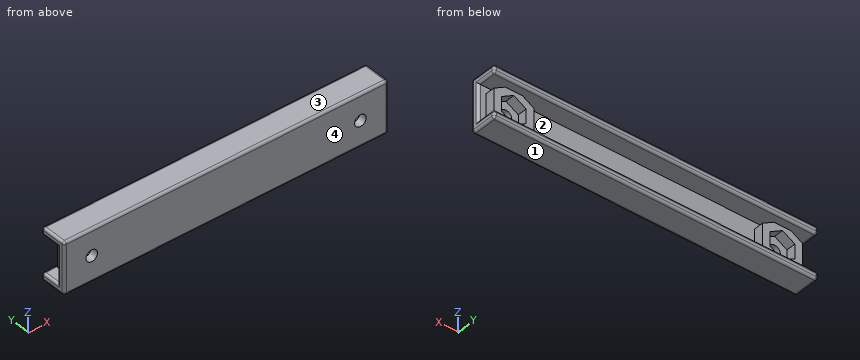
Autodesk Inventor part; units mm, degrees
ref_plane "YZ Plane" through (0, 0, 0) normal (1, 0, 0) x (0, 1, 0)
ref_plane "XZ Plane" through (0, 0, 0) normal (0, 1, 0) x (-1, 0, 0)
ref_plane "XY Plane" through (0, 0, 0) normal (0, 0, 1) x (1, 0, 0)
sketch "Sketch1" plane through (0, 0, 0) normal (0, 1, 0) x (-1, 0, 0)
  line L0 (0, 0) -> (107.315, 0)
  line L1 (107.315, 0) -> (107.315, -17.145)
  line L2 (107.315, 0) -> (124.46, 0) construction
  line L3 (107.315, -17.145) -> (0, -17.145)
  line L4 (0, -17.145) -> (0, 0)
  dimension "d0" = 107.315
  dimension "d1" = 17.145
  dimension "d2" = 90
extrude "Extrusion1" add sketch "Sketch1" along normal blind 2.54
sketch "Sketch2" plane through (0, 2.54, 0) normal (0, 1, 0) x (1, 0, 0)
  line L0 (0, 0) -> (0, 17.145)
  line L1 (0, 8.5725) -> (-9.2075, 8.5725) construction
  line L2 (0, 8.5725) -> (-2.576, 8.5725)
  line L3 (-2.576, 8.5725) -> (-2.576, 12.4012)
  line L4 (-2.576, 8.5725) -> (-2.576, 4.7438)
  line L5 (0, 17.145) -> (0, 14.605)
  line L6 (0, 14.605) -> (-107.315, 14.605)
  line L7 (-107.315, 17.145) -> (-107.315, 0)
  line L8 (-107.315, 14.605) -> (-107.315, 17.145)
  line L9 (0, 17.145) -> (-107.315, 17.145)
  line L10 (-107.315, 17.145) -> (0, 17.145)
  line L11 (0, 0) -> (0, 2.54)
  line L12 (0, 2.54) -> (-107.315, 2.54)
  line L13 (-107.315, 0) -> (0, 0)
  line L14 (-2.576, 12.4012) -> (-6.3932, 14.605)
  line L15 (-6.3932, 14.605) -> (-12.032, 14.605)
  line L16 (-2.576, 4.7438) -> (-6.3932, 2.54)
  line L17 (-12.032, 14.605) -> (-15.839, 12.4071)
  line L18 (-15.839, 12.4071) -> (-15.839, 4.7438)
  line L19 (-15.839, 4.7438) -> (-12.0218, 2.54)
  line L20 (-9.2075, 13.2969) -> (-5.116, 10.9347)
  line L21 (-5.116, 10.9347) -> (-5.116, 6.2103)
  line L22 (-5.116, 6.2103) -> (-9.2075, 3.8481)
  line L23 (-9.2075, 3.8481) -> (-13.299, 6.2103)
  line L24 (-13.299, 6.2103) -> (-13.299, 10.9347)
  line L25 (-13.299, 10.9347) -> (-9.2075, 13.2969)
  line L26 (-53.6575, 14.605) -> (-53.6575, 2.54) construction
  line L27 (-107.315, 8.5725) -> (-98.1075, 8.5725) construction
  line L28 (-107.315, 8.5725) -> (-104.739, 8.5725)
  line L29 (-104.739, 8.5725) -> (-104.739, 12.4012)
  line L30 (-104.739, 8.5725) -> (-104.739, 4.7438)
  line L31 (-104.739, 12.4012) -> (-100.9218, 14.605)
  line L32 (-104.739, 4.7438) -> (-100.9218, 2.54)
  line L33 (-95.283, 14.605) -> (-91.476, 12.4071)
  line L34 (-91.476, 12.4071) -> (-91.476, 4.7438)
  line L35 (-91.476, 4.7438) -> (-95.2932, 2.54)
  line L36 (-98.1075, 8.5725) -> (-98.1075, 14.605)
  line L37 (-98.1075, 13.2969) -> (-102.199, 10.9347)
  line L38 (-102.199, 10.9347) -> (-102.199, 6.2103)
  line L39 (-102.199, 6.2103) -> (-98.1075, 3.8481)
  line L40 (-98.1075, 3.8481) -> (-94.016, 6.2103)
  line L41 (-94.016, 6.2103) -> (-94.016, 10.9347)
  line L42 (-94.016, 10.9347) -> (-98.1075, 13.2969)
  line L43 (-100.9218, 14.605) -> (-95.283, 14.605)
  line L44 (-100.9218, 2.54) -> (-95.2932, 2.54)
  point P0 (-8.3776, 2.54)
  point P1 (-9.2075, 14.605)
  dimension "d5" = 9.2075
  dimension "d16" = 2.54
  dimension "d17" = 90
  dimension "d18" = 2.54
  dimension "d20" = 5.6388
  dimension "d30" = 4.7244
  dimension "d43" = 2.54
  dimension "d44" = 2.54
  dimension "d45" = 2.54
  dimension "d46" = 2.54
hole "Hole1" at (-9.2075, 2.54, -8.5725) direction (0, -1, 0) diameter 3.81 end through all
extrude "Extrusion2" add sketch "Sketch2" along normal blind 6.35 contours L13 L7 L12 L0 | L6 L7 L9 L0
extrude "Extrusion4" add sketch "Sketch2" along normal blind 3.175 contours L12 L19 L18 L17 L6 L14 L3 L4 L16 | L32 L30 L29 L31 L6 L33 L34 L35 L12
hole "Hole2" at (-98.1075, 2.54, -8.5725) direction (0, -1, 0) diameter 3.81 end through all
fillet "Fillet1" radius 0.7874 22 edges at (-107.315, 0, -8.5725) (-53.6575, 0, 0) (-53.6575, 0, -17.145) (0, 0, -8.5725) (-107.315, 4.445, -17.145) (-107.315, 5.715, -14.605) (-107.315, 2.54, -8.5725) (-107.315, 5.715, -2.54) (-107.315, 4.445, 0) (-107.315, 8.89, -1.27) (-107.315, 8.89, -15.875) (-53.6575, 8.89, -17.145) (-53.6575, 8.89, -14.605) (-53.6575, 8.89, -2.54) (-53.6575, 8.89, 0) (0, 8.89, -1.27) (0, 4.445, 0) (0, 5.715, -2.54) (0, 2.54, -8.5725) (0, 5.715, -14.605) (0, 4.445, -17.145) (0, 8.89, -15.875)
equation "\"BendRadius\" = Thickness"
equation "\"BendReliefWidth\" = Thickness"
equation "\"BendReliefDepth\" = 0.5 * Thickness"
equation "\"CornerReliefSize\" = 4 * Thickness"
equation "\"MinimumRemnant\" = 2 * Thickness"
equation "\"TransitionRadius\" = BendRadius"
equation "\"JacobiRadiusSize\" = Thickness"
equation "\"GapSize\" = Thickness"
properties part number "LiDAR_mount_sweepclamp_Rev.1"
Work out the finished part from the listing and answer in its coordinate system (mm). Face numbers are marked on the shaded views. Coordinates: 2 decimals unless noted, no trailing zeros. Loops run counter-clockwise (first coordinate to the right, second up) from the corner with the lowest first, then second, coordinate; pieces in that order, holes last. Notation, with made-up numbers: (-8.75, -40) - (1.25, -40) arc R11 ccw to (1.25, -35) - close; hole circle Ø7 at (-12.75, 21.25). An arc over 180 degrees is marked (long way). Use a Markdown table: item, result.
Item 1: The mould has two halves that part along Z. Classify the marked faces 1, 2, 3 and 4: +Z half, -Z half, draft (parallel to the pull), parting line (faces both ways), or undercut.
Evaluation:
| item | result |
|---|---|
| face 1 | -Z half |
| face 2 | undercut |
| face 3 | +Z half |
| face 4 | draft |
Item 2: Consider probe 1 along X at (y, z) = (5, -9.5); probe 2 along Z at (x, y) = (-47.5, 5.5) (3 decimals); probe 3 along X at (y, z) = (3.5, -11.5). Determine where each line is inside the solid, lowest interval first. Write a range as from..to.
Evaluation:
| item | result |
|---|---|
| probe 1 | x = -104.74..-102.2, -94.02..-91.48, -15.84..-13.3, -5.12..-2.58 |
| probe 2 | z = -17.145..-14.605, -2.54..0 |
| probe 3 | x = -104.74..-101.22, -95..-91.48, -15.84..-12.32, -6.1..-2.58 |
Item 3: Find section A-A, the plane y = 7. Determine the outline of the cut face in (x, z) (3 decimals).
Evaluation:
| item | result |
|---|---|
| outline | (-107.315, -16.358) arc R0.787 ccw to (-106.528, -17.145) - (-0.787, -17.145) arc R0.787 ccw to (0, -16.358) - (0, -15.392) arc R0.787 ccw to (-0.787, -14.605) - (-106.528, -14.605) arc R0.787 ccw to (-107.315, -15.392) - close; (-107.315, -1.753) arc R0.787 ccw to (-106.528, -2.54) - (-0.787, -2.54) arc R0.787 ccw to (0, -1.753) - (0, -0.787) arc R0.787 ccw to (-0.787, 0) - (-106.528, 0) arc R0.787 ccw to (-107.315, -0.787) - close |
Item 4: Find section B-B, the plane x = -44.5. Determine the outline of the cut face in (y, z) (3 decimals), and give its area (3 significant figures).
Evaluation:
| item | result |
|---|---|
| outline | (0, -16.358) arc R0.787 ccw to (0.787, -17.145) - (8.103, -17.145) arc R0.787 ccw to (8.89, -16.358) - (8.89, -15.392) arc R0.787 ccw to (8.103, -14.605) - (2.54, -14.605) - (2.54, -2.54) - (8.103, -2.54) arc R0.787 ccw to (8.89, -1.753) - (8.89, -0.787) arc R0.787 ccw to (8.103, 0) - (0.787, 0) arc R0.787 ccw to (0, -0.787) - close |
| area | 75.0 mm2 |
Item 5: Given pin 1 Ø1.6 at (y, z) = (4.5, -9) entering from -X; pin 2 Ø3.5 at (y, z) = (4, -8) entering from -X; pin 3 Ø1.6 at (y, z) = (4.5, -8.5) entering from +X, each flat-ended and moving along its own axis, determine where each tip first touches the part or whether it passes through.
Evaluation:
| item | result |
|---|---|
| pin 1 | stops at x = -104.74 |
| pin 2 | stops at x = -107.14 |
| pin 3 | stops at x = -2.58 |
